```python
from build123d import *

# Parameters (mm, degrees)
SKETCH2_W               = 43.3
SKETCH2_H               = 71.19
SKETCH2_W_2             = 31.3
SKETCH2_H_2             = 59.19
BOSS_EXTRUDE1_DEPTH     = 5
SKETCH3_W               = 8.89
SKETCH3_H               = 6
BOSS_EXTRUDE2_DEPTH     = 8.8
CUT_EXTRUDE1_DEPTH      = 76.678124977
CUT_EXTRUDE1_DEPTH_BACK = 76.678124977
SKETCH5_R               = 2.2479
SKETCH6_R               = 1.75
SKETCH6_R_2             = 1.27
CUT_EXTRUDE2_DEPTH      = 5


with BuildPart() as part:
    # Sketch2 → Boss-Extrude1 (new body)
    with BuildSketch(Plane.XY):
        Rectangle(SKETCH2_W, SKETCH2_H)
        Rectangle(SKETCH2_W_2, SKETCH2_H_2, mode=Mode.SUBTRACT)
    extrude(amount=BOSS_EXTRUDE1_DEPTH)

    # Sketch3 → Boss-Extrude2 (add)
    with BuildSketch(Plane.XY.offset(5)):
        with Locations((0, 32.595)):
            Rectangle(SKETCH3_W, SKETCH3_H)
        with Locations((0, -32.595)):
            Rectangle(SKETCH3_W, SKETCH3_H)
    extrude(amount=BOSS_EXTRUDE2_DEPTH)

    # Sketch5 → Cut-Extrude1 (cut, two sides: drawn at the far end of the back side and taken through both)
    with BuildSketch(Plane(origin=(0, 35.595, 0), x_dir=(1, 0, 0), z_dir=(0, 1, 0)).offset(-CUT_EXTRUDE1_DEPTH_BACK)):
        with BuildLine():
            Line((-4.445, -13.8), (-2.8e-08, -13.8))
            ThreePointArc((-2.8e-08, -13.8), (-3.127220221, -12.513973022), (-4.445, -9.4))
            Line((-4.445, -9.4), (-4.445, -13.8))
        make_face()
        with BuildLine():
            Line((4.445, -13.8), (4.445, -9.4))
            ThreePointArc((4.445, -9.4), (3.127220202, -12.513973041), (-2.8e-08, -13.8))
            Line((-2.8e-08, -13.8), (4.445, -13.8))
        make_face()
        with Locations(Location((0, -9.354769886, 0), (0, 0, 90))):
            Circle(SKETCH5_R)
    extrude(amount=CUT_EXTRUDE1_DEPTH + CUT_EXTRUDE1_DEPTH_BACK, mode=Mode.SUBTRACT)

    # Sketch6 → Cut-Extrude2 (cut)
    with BuildSketch(Plane(origin=(0, 0, 0), x_dir=(-1, 0, 0), z_dir=(0, 0, -1))):
        with BuildLine():
            Line((-15.65, -2.589888065), (-17.5, -2.589888065))
            ThreePointArc((-17.5, -2.589888065), (-16.262563133, -3.102451197), (-15.75, -4.339888065))
            ThreePointArc((-15.75, -4.339888065), (-17.5, -6.089888065), (-19.25, -4.339888065))
            Line((-19.25, -4.339888065), (-19.25, -9.339888065))
            ThreePointArc((-19.25, -9.339888065), (-17.5, -7.589888065), (-15.75, -9.339888065))
            ThreePointArc((-15.75, -9.339888065), (-16.262563133, -10.577324932), (-17.5, -11.089888065))
            Line((-17.5, -11.089888065), (-15.65, -11.089888065))
            Line((-15.65, -11.089888065), (-15.65, -2.589888065))
        make_face()
        with Locations((-17.5, -4.339888065)):
            Circle(SKETCH6_R)
        with Locations((-17.5, -9.339888065)):
            Circle(SKETCH6_R)
        with Locations((17.5, -9.395)):
            Circle(SKETCH6_R)
        with BuildLine():
            ThreePointArc((19.25, -4.395), (16.262563133, -5.632436867), (17.5, -2.645))
            Line((17.5, -2.645), (15.65, -2.645))
            Line((15.65, -2.645), (15.65, -11.145))
            Line((15.65, -11.145), (17.5, -11.145))
            ThreePointArc((17.5, -11.145), (16.262563133, -8.157563133), (19.25, -9.395))
            Line((19.25, -9.395), (19.25, -4.395))
        make_face()
        with Locations((17.5, -4.395)):
            Circle(SKETCH6_R)
        with Locations((-18.5, 18.49499991)):
            Circle(SKETCH6_R_2)
        with Locations((18.5, 18.495)):
            Circle(SKETCH6_R_2)
        with Locations((18.5, -18.495)):
            Circle(SKETCH6_R_2)
        with Locations((-18.49999995, -18.439888065)):
            Circle(SKETCH6_R_2)
    extrude(amount=-CUT_EXTRUDE2_DEPTH, mode=Mode.SUBTRACT)


solid = part.part
```
The listing builds one solid part. Answer for the finished solid, in the listing's coordinates (mm). A direction names the side the tool comes from. Give positions to 0.01 mm unless a question says otherwise; leave off trailing zeros. Write each loop counter-clockwise with the first axis right and the second up, starting at its lowest first coordinate (ties: lowest second). Pieces come first, ordered by that corner, then holes. Notation, with made-up numbers: (14, 11.25) - (72, 11.25) arc R22 cw to (72, 48.25) - close; hole circle Ø11 at (12, 57.5). An arc over 180 degrees is marked (long way). Use one line per item in the form item = value. Start each with the question number.
1) Find section A-A on x = 8. Determine the outline of the cut face in (y, z) (3 decimals).
2) Find section B-B on y = -8. Determine the outline of the cut face in (x, z).
3) The mould has two halves that part along X. Classify faces 4 (the face through (-17, 0, 5)), 5 (the face through (-4.445, 33, 7)), 6 (the face through (-19.183, 19.566, 2.465)): pulls with the +X half, pulls with the -X half, needs draft (parallel to the pull), parting line crosses it, or undercut.
4) A tool of negligible diameter and unlimited length cuts with its end or side. For faces 1 (the face through (-0.675, 32.553, 7.211)), 2 (the face through (-15.65, 13, 2)), 3 (the face through (17, 0, 5)), from which of +Z, -Z, +X, -X, +Y, -Y can it reach the whole face along a straight path? Write none if from no direction.
5) Consider line 1 along X through (y, z) = (4, 3); line 2 along Y through (x, z) = (18.5, 2.2) (3 decimals); line 3 along Y through (x, z) = (4, 3) (3 decimals). Determine where each line is inside the solid, lowest interval first. Write a range as from..to.
6) Find section C-C on x = -18.5. Determine the outline of the cut face in (y, z) (3 decimals), plus the area to 3 significant figures.
7) Flat-ended cylindrical pins translate along their axes: pin 1 Ø1.3 at (y, z) = (33.5, 6.5) entering from +X (3 decimals); pin 2 Ø3.5 at (x, y) = (-18.5, 18.495) entering from +Z; pin 3 Ø3.5 at (y, z) = (32, 7.5) entering from -X (3 decimals). Find the tip coordinate at first contact, or state that the pin passes through.
Geometry results:
q1.outline = (-35.595, 0) - (-29.595, 0) - (-29.595, 5) - (-35.595, 5) - close; (29.595, 0) - (35.595, 0) - (35.595, 5) - (29.595, 5) - close
q2.outline = (-21.65, 0) - (-19.25, 0) - (-19.25, 5) - (-21.65, 5) - close; (19.25, 0) - (21.65, 0) - (21.65, 5) - (19.25, 5) - close
q3.face_4 = needs draft
q3.face_5 = pulls with the -X half
q3.face_6 = undercut
q4.face_1 = +Y, -Y
q4.face_2 = +Z, -Z
q4.face_3 = +Z, +X, +Y, -Y
q5.line_1 = -21.65..-15.65, 15.65..21.65
q5.line_2 = -35.595..-19.71, -17.17..-10.776, -2.904..17.225, 19.765..35.595
q5.line_3 = -35.595..-29.595, 29.595..35.595
q6.outline = (-35.595, 0) - (-19.765, 0) - (-19.765, 5) - (-35.595, 5) - close; (-17.225, 0) - (-10.831, 0) - (-10.831, 5) - (-17.225, 5) - close; (-2.959, 0) - (17.225, 0) - (17.225, 5) - (-2.959, 5) - close; (19.765, 0) - (35.595, 0) - (35.595, 5) - (19.765, 5) - close
q6.area = 291 mm2
q7.pin_1 = 4.445
q7.pin_2 = 5
q7.pin_3 = -4.445
